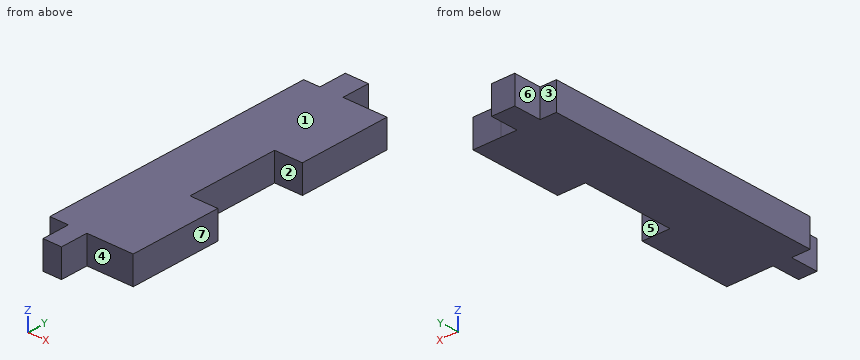
from build123d import *

# Parameters (mm, degrees)
SKETCH1_W           = 4.166666667
SKETCH1_H           = 5
SKETCH1_W_2         = 3.333333333
BOSS_EXTRUDE1_DEPTH = 5
CAVITY1_START       = -27.230031218
CAVITY1_OUTLINE_W   = 16.666666667
CAVITY1_OUTLINE_H   = 5
CAVITY1_DEPTH       = 5


# Read off the part's stored shape, not the designer's step: Cavity1
with BuildPart() as part:
    # Sketch1 → Boss-Extrude1 (new body)
    with BuildSketch(Plane.XY):
        with Locations((-32.230031219, -13.680003411)):
            Rectangle(SKETCH1_W, SKETCH1_H)
        Polygon((-34.313364552, -21.180003411), (-34.313364552, -16.180003411), (-37.230031218, -16.180003411), (-37.230031218, -66.180003411), (-33.896697885, -66.180003411), (-33.896697885, -61.180003411), (-30.563364552, -61.180003411), (-30.563364552, -66.180003411), (-27.230031218, -66.180003411), (-27.230031218, -16.180003411), (-30.146697885, -16.180003411), (-30.146697885, -21.180003411), align=None)
        with Locations((-32.230031219, -18.680003411)):
            Rectangle(SKETCH1_W, SKETCH1_H)
        Polygon((-22.230031218, -16.180335931), (-27.230031218, -16.180003411), (-27.230031218, -66.180003411), (-22.230031218, -66.180003411), align=None)
        with Locations((-32.230031219, -63.680003411)):
            Rectangle(SKETCH1_W_2, SKETCH1_H)
        with Locations((-32.230031219, -68.680003411)):
            Rectangle(SKETCH1_W_2, SKETCH1_H)
    extrude(amount=BOSS_EXTRUDE1_DEPTH)

    # Cavity1 outline → Cavity1 (cut)
    with BuildSketch(Plane.YZ.offset(CAVITY1_START)):
        with Locations((-41.180335932, 2.5)):
            Rectangle(CAVITY1_OUTLINE_W, CAVITY1_OUTLINE_H)
    extrude(amount=CAVITY1_DEPTH, mode=Mode.SUBTRACT)


solid = part.part
Can you work these out from the model? Positions are in its coordinate system, mm. Face numbers are marked on the shaded views. A direction names the side the tool comes from. Give positions to 0.01 mm unless a question says otherwise; leave off trailing zeros. Write each loop counter-clockwise with the first axis right and the second up, starting at its lowest first coordinate (ties: lowest second). Pieces come first, ordered by that corner, then holes. Notation, with made-up numbers: M 29.25,87.25 L 49.25,87.25 A17 cw 49.25,95.25 Z; hole C -6.75,-26 d1. An arc over 180 degrees is marked long. Answer in a Markdown table with one row per item. Add a question column.
Item 1: Please list where these lines run through material, in increasing order: L1, parallel to Y at x = -23.5, z = 0.9; L2, parallel to X at y = -43, z = 2.4; L3, parallel to Y at x = -35.75, z = 2.05.
Item 2: For pin 1 Ø1.5 at (x, z) = (-24, 4) entering from -Y; pin 2 Ø2.5 at (y, z) = (-69.5, 1.5) entering from +X; pin 3 Ø2.5 at (x, z) = (-25.5, 2.5) entering from +Y, each with a flat end and sliding along its axis, tell me the tip position at first contact or that it passes through.
Item 3: Imagine slicing it at B-B, the plane x = -26. Write out the boundary of the cut face in (y, z).
Item 4: Imagine slicing it at D-D, the plane x = -29.25. Write out the boundary of the cut face in (y, z).
Item 5: Imagine slicing it at A-A, the plane z = 1.4. Write out the boundary of the cut face in (x, y), plus the area to 3 significant figures.
Item 6: We'd pull the mould along Y, two halves only. Please class the marked faces 1, 2 and 3: released by +Y, released by -Y, zero draft, split by the parting line, or undercut.
Item 7: On a 3-axis mill with a long thin cutter (end or side, diameter ignored), from which of +Z, -Z, +X, -X, +Y, -Y can I reach the whole of each face in a straight line? I mean the marked faces 4, 5, 6 and 7. Say none if no direction works.
Item 8: Imagine slicing it at C-C, the plane y = -36.5. Write out the boundary of the cut face in (x, z).
Evaluation:
| question | item | result |
|---|---|---|
| 1 | L1 | y = -66.18 to -49.51, -32.85 to -16.18 |
| 1 | L2 | x = -37.23 to -27.23 |
| 1 | L3 | y = -66.18 to -16.18 |
| 2 | pin 1 | stops at y = -66.18 |
| 2 | pin 2 | stops at x = -30.56 |
| 2 | pin 3 | stops at y = -16.18 |
| 3 | outline | M -66.18,0 L -49.51,0 L -49.51,5 L -66.18,5 Z; M -32.85,0 L -16.18,0 L -16.18,5 L -32.85,5 Z |
| 4 | outline | M -66.18,0 L -16.18,0 L -16.18,5 L -66.18,5 Z |
| 5 | outline | M -37.23,-66.18 L -33.9,-66.18 L -33.9,-71.18 L -30.56,-71.18 L -30.56,-66.18 L -22.23,-66.18 L -22.23,-49.51 L -27.23,-49.51 L -27.23,-32.85 L -22.23,-32.85 L -22.23,-16.18 L -27.23,-16.18 L -30.15,-16.18 L -30.15,-11.18 L -34.31,-11.18 L -34.31,-16.18 L -37.23,-16.18 Z |
| 5 | area | 704 mm² |
| 6 | face 1 | zero draft |
| 6 | face 2 | undercut |
| 6 | face 3 | released by +Y |
| 7 | face 4 | +Z, -Z, +X, -Y |
| 7 | face 5 | +Z, -Z, +X |
| 7 | face 6 | +Z, -Z, -X, +Y |
| 7 | face 7 | +Z, -Z, +X, +Y, -Y |
| 8 | outline | M -37.23,0 L -27.23,0 L -27.23,5 L -37.23,5 Z |
